Print and shaded views of the part. All mm, measured from the part's lowest x, y and z. Round coordinates to 2 decimals unless told otherwise and drop trailing zeros. Loops run counter-clockwise (first coordinate to the right, second up) from the corner with the lowest first, then second, coordinate; pieces in that order, holes last. Notation, with made-up numbers: (51, 55.25) - (83, 55.25) arc R23 ccw to (83, 63.25) - close; hole circle Ø5 at (8, 2.5). An arc over 180 degrees is marked (long way). Answer as a JSON object with one key per item and string values.
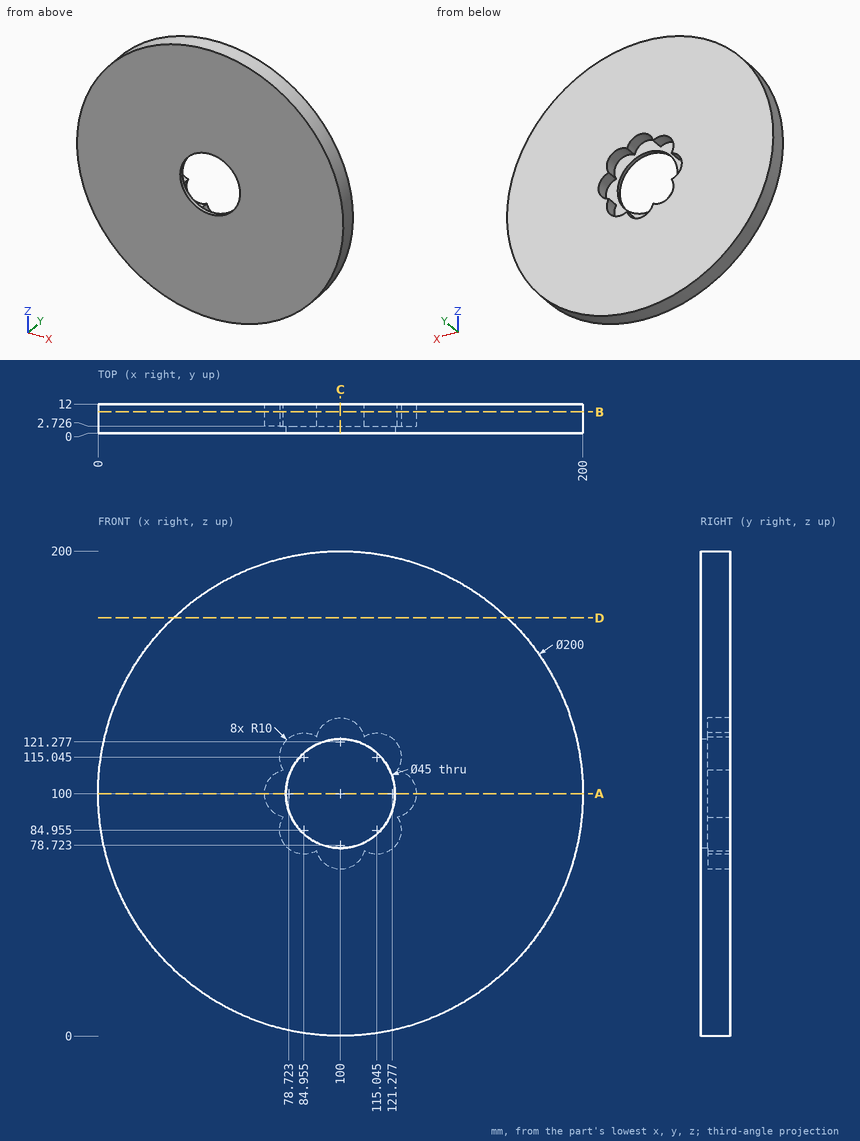
1) Slice it at C-C on x = 100. List the corners of the cut face in (y, z).
Values follow:
{"outline": "(0, 0) - (12, 0) - (12, 68.72) - (2.73, 68.72) - (2.73, 77.5) - (0, 77.5) - close; (0, 122.5) - (2.73, 122.5) - (2.73, 131.28) - (12, 131.28) - (12, 200) - (0, 200) - close"}
2) Slice it at B-B on y = 8.75. List the corners of the cut face in (x, z) (1 decimal).
Values follow:
{"outline": "circle Ø200 at (100, 100); hole (76.5, 90.3) arc R10 ccw to (90.3, 76.5) arc R10 ccw to (109.7, 76.5) arc R10 ccw to (123.5, 90.3) arc R10 ccw to (123.5, 109.7) arc R10 ccw to (109.7, 123.5) arc R10 ccw to (90.3, 123.5) arc R10 ccw to (76.5, 109.7) arc R10 ccw to start"}
3) Drop flat-ended pins along their axis: P1, Ø5, axis at y = 1.5, z = 137, coming from the +X side; P2, Ø6, axis at y = 4.5, z = 88, coming from the -X side; P3, Ø1, axis at y = 5.5, z = 148.5, coming from the +X side. Give the stop position or say it passes through.
Values follow:
{"P1": "x = 193.86", "P2": "x = 0.41", "P3": "x = 187.73"}
4) Probe probe 1 along X at (y, z) = (0.8, 100); probe 2 along Z at (x, y) = (79.5, 5.25) (1 decimal); probe 3 along Z at (x, y) = (98, 11) (1 decimal). List the from-to ranges inside material, lowest first.
Values follow:
{"probe 1": "0 to 77.5, 122.5 to 200", "probe 2": "2.1 to 76.6, 123.4 to 197.9", "probe 3": "0 to 68.9, 131.1 to 200"}
5) Slice it at A-A on z = 100. List the corners of the cut face in (x, y), then the cut area to 3 significant figures.
Values follow:
{"outline": "(0, 0) - (77.5, 0) - (77.5, 2.73) - (68.72, 2.73) - (68.72, 12) - (0, 12) - close; (122.5, 0) - (200, 0) - (200, 12) - (131.28, 12) - (131.28, 2.73) - (122.5, 2.73) - close", "area": "1,700 mm²"}
6) Slice it at D-D on z = 172.5. List the corners of the cut face in (x, y) (1 decimal), then the cut area to 3 significant figures.
Values follow:
{"outline": "(31.1, 0) - (168.9, 0) - (168.9, 12) - (31.1, 12) - close", "area": "1,650 mm²"}
